Source: three-view drawing plus pictorial views. Frame: mm from the lowest corner of the part. A direction names the side the tool comes from. Give positions to 0.01 mm unless a question says otherwise; leave off trailing zeros. Loops run counter-clockwise (first coordinate to the right, second up) from the corner with the lowest first, then second, coordinate; pieces in that order, holes last. Notation, with made-up numbers: (71, -11) -> (90, -11) arc R13 cw to (90, 1) -> close; hole circle Ø11 at (55.5, 35.5). An arc over 180 degrees is marked (long way). One line per item, written item: value. Start each with the question number.
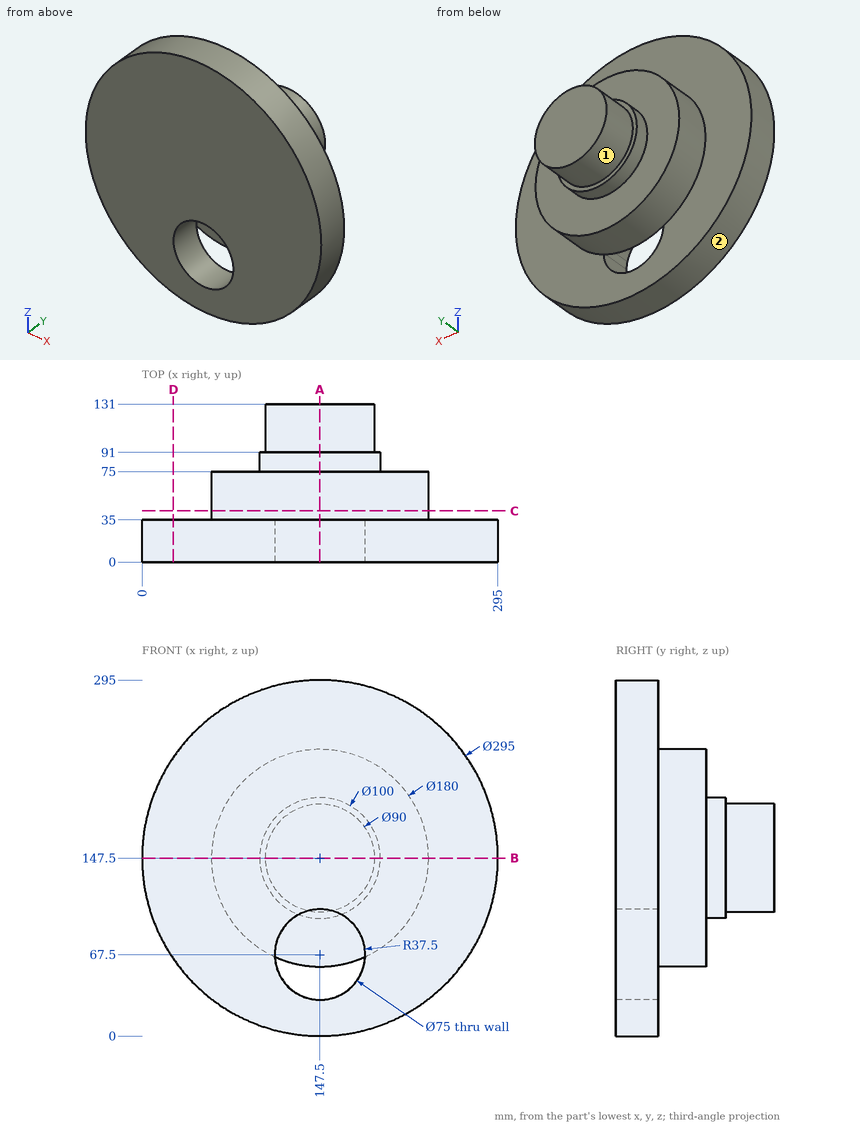
Item 1: Section D-D, the plane x = 26. Output: boundary loops of the cut face in (y, z), then the cut area to 3 significant figures.
Item 2: Section A-A, the plane x = 147.5. Output: boundary loops of the cut face in (y, z), then the cut area to 3 significant figures.
Item 3: Section B-B, the plane z = 147.5. Output: boundary loops of the cut face in (x, y).
Item 4: Ray query, line 1 along Z through (x, y) = (147.5, 13); line 2 along Y through (x, z) = (188, 77); line 3 along Y through (x, z) = (65, 230.5). Return the intervals inside material, ascending. Write a range as [from, to].
Item 5: Pin query (flat end, axial travel): pin 1 (1 mm diameter, centred on x = 179.5, z = 67, fed in from +Y); pin 2 (1.5 mm diameter, centred on x = 227.5, y = 69, fed in from +Z); pin 3 (10 mm diameter, centred on x = 257, z = 50, fed in from +Y). Return the tip coordinate at first contact, or that it passes through.
Item 6: Section C-C, the plane y = 42.5. Output: boundary loops of the cut face in (x, z).
Item 7: Access query for the marked faces 1 and 2. Directions: +Z, -Z, +X, -X, +Y, -Y. A direction counts if a zero-diameter tool reaches every point of the face in a straight line with its end or side. Return the directions, or none.
Geometry check:
1. outline: (0, 63.87) -> (35, 63.87) -> (35, 231.13) -> (0, 231.13) -> close
1. area: 5,850 mm2
2. outline: (0, 0) -> (35, 0) -> (35, 30) -> (0, 30) -> close; (0, 105) -> (35, 105) -> (35, 57.5) -> (75, 57.5) -> (75, 97.5) -> (91, 97.5) -> (91, 102.5) -> (131, 102.5) -> (131, 192.5) -> (91, 192.5) -> (91, 197.5) -> (75, 197.5) -> (75, 237.5) -> (35, 237.5) -> (35, 295) -> (0, 295) -> close
2. area: 20,100 mm2
3. outline: (0, 0) -> (295, 0) -> (295, 35) -> (237.5, 35) -> (237.5, 75) -> (197.5, 75) -> (197.5, 91) -> (192.5, 91) -> (192.5, 131) -> (102.5, 131) -> (102.5, 91) -> (97.5, 91) -> (97.5, 75) -> (57.5, 75) -> (57.5, 35) -> (0, 35) -> close
4. line 1: z = [0, 30], [105, 295]
4. line 2: y = [0, 75]
4. line 3: y = [0, 35]
5. pin 1: stops at y = 75
5. pin 2: stops at z = 190.15
5. pin 3: stops at y = 35
6. outline: circle Ø180 at (147.5, 147.5)
7. face 1: +Y
7. face 2: +Y, -Y
